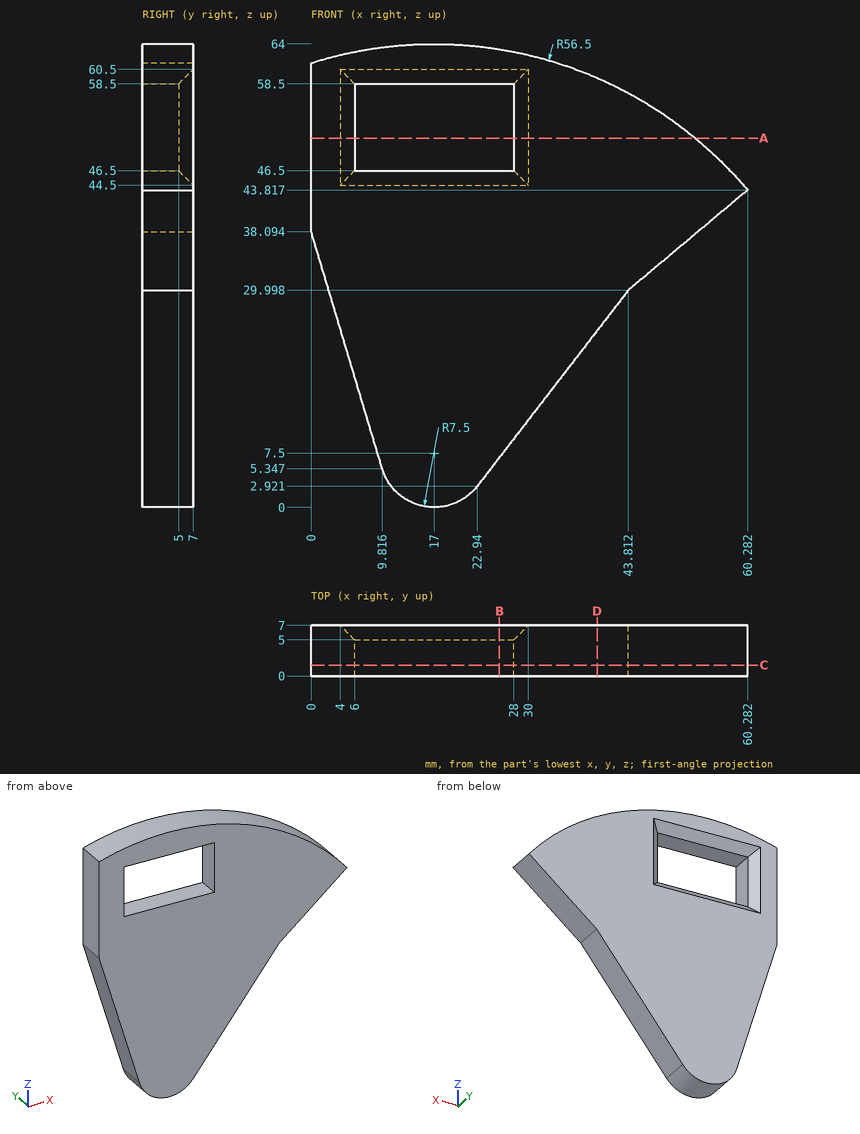
Geometry check sheet. Reference: drawing and pictorial views, mm from the part's lowest x, y, z. Coordinates: 2 decimals unless noted, no trailing zeros. Write each loop counter-clockwise with the first axis right and the second up, starting at its lowest first coordinate (ties: lowest second). Pieces come first, ordered by that corner, then holes. Notation, with made-up numbers: (31.25, -24.75) -> (79.25, -24.75) arc R10 cw to (79.25, -19.75) -> close; hole circle Ø10 at (37, 12.5). An arc over 180 degrees is marked (long way). Use a Markdown table: item, result.
1. Scan lines: line 1 along X through (y, z) = (1, 55) (1 decimal); line 2 along Z through (x, y) = (13, 6) (1 decimal); line 3 along X through (y, z) = (3.75, 39). Record each from-to range of solid material in increasing order.
Reported:
| item | result |
|---|---|
| line 1 | x = 0 to 6, 28 to 47.6 |
| line 2 | z = 1.2 to 45.5, 59.5 to 63.9 |
| line 3 | x = 0 to 54.54 |
2. Sectioned sample at D-D (x = 39.5). Enter the section's corners in (y, z) (1 decimal).
Reported:
| item | result |
|---|---|
| outline | (0, 24.4) -> (7, 24.4) -> (7, 59.3) -> (0, 59.3) -> close |
3. Sectioned sample at C-C (y = 1.5). Enter the section's corners in (x, z) (1 decimal), plus the area to 3 significant figures.
Reported:
| item | result |
|---|---|
| outline | (0, 38.1) -> (9.8, 5.3) arc R7.5 ccw to (22.9, 2.9) -> (43.8, 30) -> (60.3, 43.8) arc R56.5 ccw to (0, 61.4) -> close; hole (6, 46.5) -> (28, 46.5) -> (28, 58.5) -> (6, 58.5) -> close |
| area | 2,130 mm2 |
4. Sectioned sample at A-A (z = 51). Enter the section's corners in (x, y) (1 decimal).
Reported:
| item | result |
|---|---|
| outline | (0, 0) -> (6, 0) -> (6, 5) -> (4, 7) -> (0, 7) -> close; (28, 0) -> (53.1, 0) -> (53.1, 7) -> (30, 7) -> (28, 5) -> close |
5. Go/stop test with flat-tipped pins: pin 1 Ø2.5 at (y, z) = (2, 54) entering from +X (1 decimal); pin 2 Ø2 at (y, z) = (2, 57) entering from +X (1 decimal); pin 3 Ø1 at (y, z) = (4, 21.5) entering from -X (1 decimal). Record where each tip stops, or that it passes through.
Reported:
| item | result |
|---|---|
| pin 1 | stops at x = 50.8 |
| pin 2 | stops at x = 46 |
| pin 3 | stops at x = 4.8 |
6. Sectioned sample at B-B (x = 26). Enter the section's corners in (y, z), plus the area to 3 significant figures.
Reported:
| item | result |
|---|---|
| outline | (0, 6.89) -> (7, 6.89) -> (7, 44.5) -> (5, 46.5) -> (0, 46.5) -> close; (0, 58.5) -> (5, 58.5) -> (7, 60.5) -> (7, 63.28) -> (0, 63.28) -> close |
| area | 307 mm2 |
